from build123d import *

# Parameters (mm, degrees)
BOSS_EXTRUDE1_DEPTH = 0.75


with BuildPart() as part:
    # Sketch1 → Boss-Extrude1 (new, symmetric)
    with BuildSketch(Plane.XY):
        with BuildLine():
            Line((51.25, 0), (-51.25, 0))
            Line((-51.25, 0), (-51.25, 65))
            Line((-51.25, 65), (-43.56102042, 65))
            ThreePointArc((-43.56102042, 65), (0, 40.75), (43.56102042, 65))
            Line((43.56102042, 65), (51.25, 65))
            Line((51.25, 65), (51.25, 0))
        make_face()
    extrude(amount=BOSS_EXTRUDE1_DEPTH, both=True)


solid = part.part
Verification items for the finished model (mm, model axes). Coordinates: 2 decimals unless noted, no trailing zeros. Loops run counter-clockwise (first coordinate to the right, second up) from the corner with the lowest first, then second, coordinate; pieces in that order, holes last. Notation, with made-up numbers: M 51.25,12.25 L 87.25,12.25 A4 ccw 87.25,16.25 Z; hole C 71.25,76.25 d4. An arc over 180 degrees is marked long. One line per item, written item: value.
1. Material ranges on line 1 along X through (y, z) = (59.5, -0.5); line 2 along X through (y, z) = (58.5, 0.1); line 3 along Y through (x, z) = (-1.5, -0.3), recorded low to high. Write a range as from..to.
Answers follow:
line 1: -51.25..-39.63, 39.63..51.25
line 2: -51.25..-38.79, 38.79..51.25
line 3: 0..40.77
2. Section check A-A on y = 42.5. Record the cut outline in (x, z).
Answers follow:
outline: M -51.25,-0.75 L -13.28,-0.75 L -13.28,0.75 L -51.25,0.75 Z; M 13.28,-0.75 L 51.25,-0.75 L 51.25,0.75 L 13.28,0.75 Z
3. Section check C-C on x = 39. Record the cut outline in (y, z), plus the area to 3 significant figures.
Answers follow:
outline: M 0,-0.75 L 58.75,-0.75 L 58.75,0.75 L 0,0.75 Z
area: 88.1 mm^2
4. Section check B-B on z = 0.05. Record the cut outline in (x, y), plus the area to 3 significant figures.
Answers follow:
outline: M -51.25,0 L 51.25,0 L 51.25,65 L 43.56,65 A51.25 cw -43.56,65 L -51.25,65 Z
area: 5,170 mm^2
5. Mould release check, pull along X, two halves, no side actions. Record for faces 1 (the flat face through (1, 26, 0.75)), 2 (the cylindrical face through (-0.729, 40.755, 0.01)): pulls with the +X half, pulls with the -X half, needs draft (parallel to the pull), parting line crosses it, or undercut.
Answers follow:
face 1: needs draft
face 2: undercut
6. Section check D-D on y = 56. Record the cut outline in (x, z), plus the area to 3 significant figures.
Answers follow:
outline: M -51.25,-0.75 L -36.48,-0.75 L -36.48,0.75 L -51.25,0.75 Z; M 36.48,-0.75 L 51.25,-0.75 L 51.25,0.75 L 36.48,0.75 Z
area: 44.3 mm^2
